Part model, mm, in its own coordinate system. A direction names the side the tool comes from. Give positions to 0.01 mm unless a question says otherwise; leave off trailing zeros. Order: outer loops, then holes, each group sorted by start corner. A loop starts at its lowest first (then second) coordinate and runs counter-clockwise, first axis right, second up. Notation, with made-up numbers: M 53,17.5 L 92,17.5 A6 ccw 92,25.5 Z; hole C 89.25,86 d8. An arc over 180 degrees is marked long. Answer as a JSON object with one key per item and string values.
from build123d import *

# Parameters (mm, degrees)
F0_R     = 3
F1_DEPTH = 3.5
F2_R     = 2.15
F3_DEPTH = 2.7
F4_R     = 3.5
F5_DEPTH = 6.6
F6_R     = 4.75
F7_DEPTH = 8
F8_W     = 4
F8_H     = 0.4
F9_DEPTH = 8


with BuildPart() as f1:
    # F0 (on Top) → F1 (new body)
    with BuildSketch(Plane.XY):
        Circle(F0_R)
    extrude(amount=F1_DEPTH)

    # F2 (on face) → F3 (join)
    with BuildSketch(Plane.XY.offset(3.5)):
        Circle(F2_R)
    extrude(amount=F3_DEPTH)

    # F4 (on face) → F5 (join)
    with BuildSketch(Plane.XY.offset(6.2)):
        Circle(F4_R)
    extrude(amount=F5_DEPTH)

    # F6 (on face) → F7 (join)
    with BuildSketch(Plane.XY.offset(12.8)):
        Circle(F6_R)
    extrude(amount=F7_DEPTH)

    # F8 (on face) → F9 (join)
    with BuildSketch(Plane.XY.offset(20.8)):
        with Locations((0, -1.75)):
            Rectangle(F8_W, F8_H)
        with Locations((0, 1.75)):
            Rectangle(F8_W, F8_H)
    extrude(amount=F9_DEPTH)


solid = f1.part
1. Cut at D-D on y = 0. Give the cut face in (x, z), plus the area to 3 significant figures.
Worked answers:
{"outline": "M -4.75,12.8 L -3.5,12.8 L -3.5,6.2 L -2.15,6.2 L -2.15,3.5 L -3,3.5 L -3,0 L 3,0 L 3,3.5 L 2.15,3.5 L 2.15,6.2 L 3.5,6.2 L 3.5,12.8 L 4.75,12.8 L 4.75,20.8 L -4.75,20.8 Z", "area": "155 mm^2"}
2. Probe line 1 along Z through (x, y) = (-2.5, 4); line 2 along Z through (x, y) = (2, 1); line 3 along Z through (x, y) = (-1.5, -3). List the from-to ranges inside material, lowest first.
Worked answers:
{"line 1": "z = 12.8 to 20.8", "line 2": "z = 0 to 3.5, 6.2 to 20.8", "line 3": "z = 6.2 to 20.8"}
3. Cut at A-A on y = 2.5. Give the cut face in (x, z), plus the area to 3 significant figures.
Worked answers:
{"outline": "M -4.04,12.8 L -2.45,12.8 L -2.45,6.2 L 2.45,6.2 L 2.45,12.8 L 4.04,12.8 L 4.04,20.8 L -4.04,20.8 Z; M -1.66,0 L 1.66,0 L 1.66,3.5 L -1.66,3.5 Z", "area": "109 mm^2"}
4. Cut at C-C on x = 0. Give the cut face in (y, z).
Worked answers:
{"outline": "M -4.75,12.8 L -3.5,12.8 L -3.5,6.2 L -2.15,6.2 L -2.15,3.5 L -3,3.5 L -3,0 L 3,0 L 3,3.5 L 2.15,3.5 L 2.15,6.2 L 3.5,6.2 L 3.5,12.8 L 4.75,12.8 L 4.75,20.8 L 1.95,20.8 L 1.95,28.8 L 1.55,28.8 L 1.55,20.8 L -1.55,20.8 L -1.55,28.8 L -1.95,28.8 L -1.95,20.8 L -4.75,20.8 Z"}
5. Which spindle directions (+Z, -Z, +X, -X, +Y, -Y) get a long thin tool onto all of the face, cutting with end or side? Do faces 1 (the cylindrical face through (3.233, -1.341, 9.454)), 2 (the flat face through (0, -1.95, 25)), 3 (the flat face through (-2, -2, 6.2)), 4 (the cylindrical face through (2.192, -4.214, 16.744)), 5 (the flat face through (0, 1.55, 25)). Say none if no direction does.
Worked answers:
{"face 1": "-Z", "face 2": "+Z, +X, -X, -Y", "face 3": "none", "face 4": "+Z, -Z", "face 5": "+Z, +X, -X"}
6. Pin check, flat tips, straight feed: P1, Ø5, axis at y = -0.5, z = 26, coming from the +X side; P2, Ø4.5, axis at x = 0, z = 25.5, coming from the -Y side; P3, Ø1.8, axis at x = -1, y = -1, coming from the +Z side; P4, Ø2, axis at x = 1, z = 26.5, coming from the +Y side. Stop position of each tip, or through.
Worked answers:
{"P1": "stops at x = 2", "P2": "stops at y = -1.95", "P3": "stops at z = 28.8", "P4": "stops at y = 1.95"}
7. Cut at B-B on z = 27. Give the cut face in (x, y).
Worked answers:
{"outline": "M -2,-1.95 L 2,-1.95 L 2,-1.55 L -2,-1.55 Z; M -2,1.55 L 2,1.55 L 2,1.95 L -2,1.95 Z"}
8. Two-plate mould, pull along Z, no slides. Class faces 6 (the flat face through (-4, 0, 12.8)), 7 (the flat face through (0, 1.95, 25)), 8 (the flat face through (1.3, -2, 3.5)): +Z half, -Z half, draft (parallel to the pull), parting line (faces both ways), or undercut.
Worked answers:
{"face 6": "-Z half", "face 7": "draft", "face 8": "undercut"}
